Check sheet for the modelled part. Datum: model origin and axes. Units: mm. A direction names the side the tool comes from. Give positions to 0.01 mm unless a question says otherwise; leave off trailing zeros. Order: outer loops, then holes, each group sorted by start corner. A loop starts at its lowest first (then second) coordinate and runs counter-clockwise, first axis right, second up.
from build123d import *

# Parameters (mm, degrees)
SKETCH2_W                  = 46
SKETCH2_H                  = 28
SKETCH2_W_2                = 14
SKETCH2_H_2                = 14
BOSS_EXTRUDE1_DEPTH        = 3
F_2_6_2_6_DIAMETER_HOLE1_D = 2.6
SKETCH2_6_R                = 2.5
SKETCH2_6_W                = 20
SKETCH2_6_H                = 20
CUT_EXTRUDE2_DEPTH         = 1.5
FILLET1_R                  = 3
CUT_EXTRUDE3_DEPTH         = 0.4


with BuildPart() as part:
    # Sketch2 → Boss-Extrude1 (new body)
    with BuildSketch(Plane(origin=(0, 0, 0), x_dir=(0, 1, 0), z_dir=(0, 0, 1))):
        Rectangle(SKETCH2_W, SKETCH2_H)
        with Locations((-1, 0)):
            Rectangle(SKETCH2_W_2, SKETCH2_H_2, mode=Mode.SUBTRACT)
    extrude(amount=BOSS_EXTRUDE1_DEPTH)

    # 2.6 _2.6_ Diameter Hole1 (through all)
    with Locations(Plane(origin=(0, 0, 0), x_dir=(-1, 0, 0), z_dir=(0, 0, -1))):
        with Locations((-9, -18), (9, -18), (-9, 18), (9, 18)):
            Hole(F_2_6_2_6_DIAMETER_HOLE1_D / 2)

    # Sketch2_6 → Cut-Extrude2 (cut)
    with BuildSketch(Plane(origin=(0, 0, 0), x_dir=(0, 1, 0), z_dir=(0, 0, 1))):
        with Locations(Location((-18, -9, 0), (0, 0, 270))):
            Circle(SKETCH2_6_R)
        with Locations(Location((-18, 9, 0), (0, 0, 270))):
            Circle(SKETCH2_6_R)
        with Locations(Location((18, 9, 0), (0, 0, 270))):
            Circle(SKETCH2_6_R)
        with Locations(Location((18, -9, 0), (0, 0, 270))):
            Circle(SKETCH2_6_R)
        with Locations((-1, 0)):
            Rectangle(SKETCH2_6_W, SKETCH2_6_H)
    extrude(amount=CUT_EXTRUDE2_DEPTH, mode=Mode.SUBTRACT)

    # Fillet1
    fillet1_edges = [part.edges().sort_by_distance(p)[0] for p in [
        (-14, 23, 1.5),
        (14, 23, 1.5),
        (14, -23, 1.5),
        (-14, -23, 1.5),
    ]]
    fillet(fillet1_edges, radius=FILLET1_R)

    # Sketch6 → Cut-Extrude3 (cut)
    with BuildSketch(Plane(origin=(0, 0, 0), x_dir=(1, 0, 0), z_dir=(0, 0, -1))):
        with BuildLine():
            Line((0.5, 15), (0.5, 13))
            ThreePointArc((0.5, 13), (0, 12.5), (-0.5, 13))
            Line((-0.5, 13), (-0.5, 15))
            ThreePointArc((-0.5, 15), (0, 15.5), (0.5, 15))
        make_face()
    extrude(amount=-CUT_EXTRUDE3_DEPTH, mode=Mode.SUBTRACT)


solid = part.part
1) Draft check along X on faces 4 (the face through (0, 10, 0)), 5 (the face through (-13.14, 22.1, 1.52)), 6 (the face through (0, 9, 1)). Enter one of: +X half, -X half, draft (parallel to the pull), parting line (faces both ways), or undercut.
Recorded:
face 4: draft
face 5: -X half
face 6: undercut
2) Section check B-B, the plane y = 2.5. Record the cut outline in (x, z), then the cut area to 3 significant figures.
Recorded:
outline: (-14, 0) - (-10, 0) - (-10, 1.5) - (-7, 1.5) - (-7, 3) - (-14, 3) - close; (7, 1.5) - (10, 1.5) - (10, 0) - (14, 0) - (14, 3) - (7, 3) - close
area: 33.0 mm2
3) Set-up check for faces 1 (the face through (10.1, -19.1, 1.5)), 2 (the face through (13.1, -22.14, 1.52)), 3 (the face through (-7, -1, 2)): record each of +Z, -Z, +X, -X, +Y, -Y from which the full face is reachable in a straight line by a thin tool's end or side.
Recorded:
face 1: -Z
face 2: +Z, -Z, +X, -Y
face 3: +Z, -Z
4) Section check A-A, the plane x = -9. Record the cut outline in (y, z), then the cut area to 3 significant figures.
Recorded:
outline: (-23, 0) - (-20.5, 0) - (-20.5, 1.5) - (-19.3, 1.5) - (-19.3, 3) - (-23, 3) - close; (-16.7, 1.5) - (-15.5, 1.5) - (-15.5, 0) - (-11, 0) - (-11, 1.5) - (9, 1.5) - (9, 0) - (15.5, 0) - (15.5, 1.5) - (16.7, 1.5) - (16.7, 3) - (-16.7, 3) - close; (19.3, 1.5) - (20.5, 1.5) - (20.5, 0) - (23, 0) - (23, 3) - (19.3, 3) - close
area: 85.2 mm2
5) Depth check by flat-ended pin: pin 1 Ø1.5 at (x, y) = (-9.5, -18) entering from -Z; pin 2 Ø0.8 at (x, y) = (0, -14.5) entering from -Z. Enter the tip coordinate at first touch or a pass-through.
Recorded:
pin 1: passes through
pin 2: stops at z = 0.4
6) Material ranges on L1, parallel to Y at x = -9, z = 2.2; L2, parallel to Y at x = 9, z = 0.45; L3, parallel to X at y = -1, z = 2.25, recorded low to high.
Recorded:
L1: y = -23 to -19.3, -16.7 to 16.7, 19.3 to 23
L2: y = -23 to -20.5, -15.5 to -11, 9 to 15.5, 20.5 to 23
L3: x = -14 to -7, 7 to 14
7) Section check C-C, the plane z = 2.3. Record the cut outline in (x, y).
Recorded:
outline: (-14, -20) arc R3 ccw to (-11, -23) - (11, -23) arc R3 ccw to (14, -20) - (14, 20) arc R3 ccw to (11, 23) - (-11, 23) arc R3 ccw to (-14, 20) - close; hole circle Ø2.6 at (-9, -18); hole circle Ø2.6 at (-9, 18); hole (-7, -8) - (7, -8) - (7, 6) - (-7, 6) - close; hole circle Ø2.6 at (9, -18); hole circle Ø2.6 at (9, 18)
8) Section check D-D, the plane x = 0. Record the cut outline in (y, z), then the cut area to 3 significant figures.
Recorded:
outline: (-23, 0) - (-15.5, 0) - (-15.5, 0.4) - (-12.5, 0.4) - (-12.5, 0) - (-11, 0) - (-11, 1.5) - (-8, 1.5) - (-8, 3) - (-23, 3) - close; (6, 1.5) - (9, 1.5) - (9, 0) - (23, 0) - (23, 3) - (6, 3) - close
area: 85.8 mm2
